Check sheet for the modelled part. Datum: model origin and axes. Units: mm. Face numbers are marked on the shaded views. A direction names the side the tool comes from. Coordinates: 2 decimals unless noted, no trailing zeros. Put each result on its own line as item: value.
```python
from build123d import *

# Parameters (mm, degrees)
FILLET1_R          = 2
SKETCH2_R          = 1.25
CUT_EXTRUDE1_DEPTH = 12.25
SKETCH3_R          = 2.5
CUT_EXTRUDE2_DEPTH = 7.25


with BuildPart() as part:
    # Sketch1 → Revolve1 (revolve)
    with BuildSketch(Plane(origin=(0, 0, 0), x_dir=(1, 0, 0), z_dir=(0, 1, 0))):
        Polygon((-1.630434783, 14.4), (7.869565217, 14.4), (10.619565217, 11.390476118), (10.619565217, 4), (14.619565217, 4), (14.619565217, 0), (13.372742768, 0), (3.071692396, 0), (3.071692396, 5.7), (-1.630434783, 5.7), align=None)
    revolve(axis=Axis((-12.391304348, 0, 0), (1, 0, 0)))

    # Fillet1
    fillet1_edges = [part.edges().sort_by_distance(p)[0] for p in [
        (14.619565217, 0, 4),
    ]]
    fillet(fillet1_edges, radius=FILLET1_R)

    # Sketch2 → Cut-Extrude1 (cut)
    with BuildSketch(Plane(origin=(10.619565217, 0, 0), x_dir=(0, 0, -1), z_dir=(1, 0, 0))):
        with Locations((0, 9)):
            Circle(SKETCH2_R)
        with Locations((6.363961031, 6.363961031)):
            Circle(SKETCH2_R)
        with Locations((9, 0)):
            Circle(SKETCH2_R)
        with Locations((6.363961031, -6.363961031)):
            Circle(SKETCH2_R)
        with Locations((0, -9)):
            Circle(SKETCH2_R)
        with Locations((-6.363961031, -6.363961031)):
            Circle(SKETCH2_R)
        with Locations((-9, 0)):
            Circle(SKETCH2_R)
        with Locations((-6.363961031, 6.363961031)):
            Circle(SKETCH2_R)
    extrude(amount=-CUT_EXTRUDE1_DEPTH, mode=Mode.SUBTRACT)

    # Sketch3 → Cut-Extrude2 (cut)
    with BuildSketch(Plane.ZY.offset(1.630434783)):
        with Locations((0, 9)):
            Circle(SKETCH3_R)
        with Locations((6.363961031, 6.363961031)):
            Circle(SKETCH3_R)
        with Locations((9, 0)):
            Circle(SKETCH3_R)
        with Locations((6.363961031, -6.363961031)):
            Circle(SKETCH3_R)
        with Locations((0, -9)):
            Circle(SKETCH3_R)
        with Locations((-6.363961031, -6.363961031)):
            Circle(SKETCH3_R)
        with Locations((-9, 0)):
            Circle(SKETCH3_R)
        with Locations((-6.363961031, 6.363961031)):
            Circle(SKETCH3_R)
    extrude(amount=-CUT_EXTRUDE2_DEPTH, mode=Mode.SUBTRACT)


solid = part.part
```
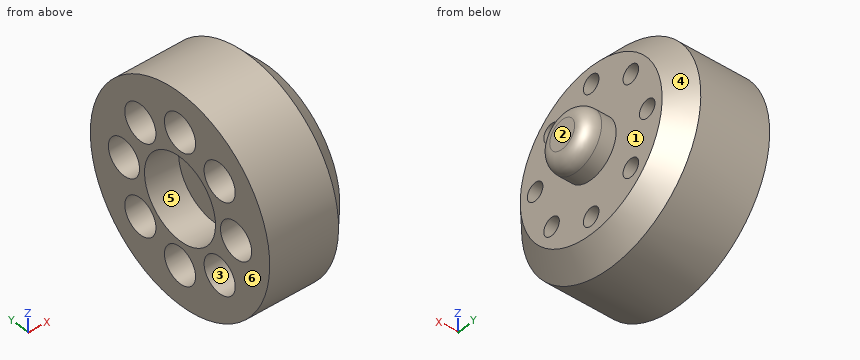
Q1. Mould release check, pull along Y, two halves, no side actions. Record for the marked faces 4, 5 and 6: released by +Y, released by -Y, zero draft, split by the parting line, or undercut.
Recorded:
face 4: split by the parting line
face 5: undercut
face 6: zero draft
Q2. Material ranges on line 1 along Y through (x, z) = (4, 0); line 2 along Y through (x, z) = (0.4, 0); line 3 along Z through (x, y) = (4.25, 0.25), recorded low to high.
Recorded:
line 1: y = -14.4 to -11.5, -6.5 to 6.5, 11.5 to 14.4
line 2: y = -14.4 to -11.5, -6.5 to -5.7, 5.7 to 6.5, 11.5 to 14.4
line 3: z = -14.4 to -11.49, -6.51 to 6.51, 11.49 to 14.4
Q3. Depth check by flat-ended pin: P1, Ø1, axis at x = 6, y = -8.5, coming from the +Z side; P2, Ø3, axis at y = 6.36, z = -6.36, coming from the +X side; P3, Ø3, axis at y = 10.5, z = -10, coming from the +X side; P4, Ø1, axis at x = 12.5, z = -9, coming from the -Y side. Enter the tip coordinate at first touch or a pass-through.
Recorded:
P1: stops at z = 11.97
P2: stops at x = 10.62
P3: stops at x = 9.15
P4: passes through
Q4. Tool access check on the marked faces 1, 2 and 3. Record the directions out of +Z, -Z, +X, -X, +Y, -Y that give a thin tool (end or side, any length) a straight path to the whole face; none if there is none.
Recorded:
face 1: +X
face 2: +Z, -Z, +X, +Y, -Y
face 3: -X
Q5. Cross-section at A-A (z = 0). State how many separate pieces and enclosed holes the cut face has, plus the area to 3 significant figures.
Recorded:
separate pieces: 3
enclosed holes: 0
area: 224 mm2
